CAD build for the part. Positions are in the model's coordinates, mm. A direction names the side the tool comes from. Give positions to 0.01 mm unless a question says otherwise; leave off trailing zeros. Loops run counter-clockwise (first coordinate to the right, second up) from the corner with the lowest first, then second, coordinate; pieces in that order, holes last.
Autodesk Inventor part; units mm, degrees
ref_plane "Arbeitsebene10" through (-35, 70.3553, 70.3553) normal (0, 1, 0) x (1, 0, 0)
ref_plane "Arbeitsebene11" through (-17.5, 90.3553, 53.0624) normal (0, 1, 0) x (1, 0, 0)
ref_plane "Arbeitsebene2" through (-35, 80.3553, 35.7696) normal (0, 1, 0) x (1, 0, 0)
ref_plane "Arbeitsebene10" through (-35, 70.3553, 70.3553) normal (0, 1, 0) x (1, 0, 0)
sketch "Skizze7" plane through (-35, 70.3553, 70.3553) normal (0, 1, 0) x (1, 0, 0)
  circle A0 centre (17.5, 17.2929) radius 11.5
  point P0 (35, 70.3553)
  dimension "d32" = 23
extrude "Achshalter" add sketch "Skizze7" along normal blind 20
ref_plane "Arbeitsebene11" through (-17.5, 90.3553, 53.0624) normal (0, 1, 0) x (1, 0, 0)
sketch "Skizze16" plane through (-17.5, 90.3553, 53.0624) normal (0, 1, 0) x (1, 0, 0)
  circle A0 centre (0, 0) radius 11.5
  arc A1 (2.2, 1.3856) -> (2.2, -1.3856) centre (0, 0) ccw
  line L0 (2.2, 1.3856) -> (2.2, -1.3856)
  point P0 (17.5, 53.0624)
  dimension "d54" = 5.2
  dimension "d55" = 2.2
extrude "Extrusion11" cut sketch "Skizze16" against normal blind 18 contours L0 A1
ref_plane "Arbeitsebene2" through (-35, 80.3553, 35.7696) normal (0, 1, 0) x (1, 0, 0)
sketch "Skizze17" plane through (-35, 80.3553, 35.7696) normal (0, 1, 0) x (1, 0, 0)
  line L0 (30.7802, -4.1446) -> (17.4658, -4.1446)
  line L1 (17.4658, -4.1446) -> (17.4658, -31.1746)
  line L2 (17.4658, -31.1746) -> (30.7802, -31.1746)
  line L3 (30.7802, -31.1746) -> (30.7802, -4.1446)
  point P0 (35, 35.7696)
extrude "Extrusion12" cut sketch "Skizze17" against normal blind 1
ref_plane "Arbeitsebene16" through (-34, 67.3553, 52.8553) normal (0, 0, 1) x (1, 0, 0)
sketch "Skizze18" plane through (-34, 67.3553, 52.8553) normal (0, 0, 1) x (1, 0, 0)
  line L0 (29.7456, 25.5785) -> (16.4577, 25.5785)
  line L1 (16.4577, 25.5785) -> (16.4577, 12.5204)
  line L2 (16.4577, 12.5204) -> (29.7456, 12.5204)
  line L3 (29.7456, 12.5204) -> (29.7456, 25.5785)
  point P0 (34, -67.3553)
extrude "Extrusion13" cut sketch "Skizze18" along normal blind 1 and the other way blind 0.5
ref_plane "Arbeitsebene17" through (-34, 67.3553, 70.3553) normal (0, 0, 1) x (1, 0, 0)
sketch "Skizze19" plane through (-34, 67.3553, 70.3553) normal (0, 0, 1) x (1, 0, 0)
  circle A0 centre (22.3096, 18.1328) radius 1.25
  point P0 (34, -67.3553)
  dimension "d67" = 2.5
extrude "Extrusion14" cut sketch "Skizze19" against normal blind 35
sketch "Skizze24" plane through (-17.5, 70.3553, 53.0624) normal (0, -1, 0) x (1, 0, 0)
  line L0 (-17.5, 17.5) -> (17.5, 17.5)
  line L1 (17.5, 17.5) -> (17.5, -17.5)
  line L2 (17.5, -17.5) -> (-17.5, -17.5)
  line L3 (-17.5, -17.5) -> (-17.5, 17.5)
  point P0 (0, 0)
  point P1 (17.5, -53.0624)
  dimension "d90" = 35
  dimension "d91" = 35
  dimension "d92" = 17.5
  dimension "d93" = 17.5
extrude "Extrusion17" add sketch "Skizze24" along normal blind 5
sketch "Skizze25" plane through (-35, 70.3553, 35.5624) normal (-1, 0, 0) x (0, 0, 1)
  line L0 (35, -5) -> (0, -5)
  line L1 (0, -5) -> (0, -40)
  line L2 (0, -40) -> (35, -40)
  line L3 (35, -40) -> (35, -5)
  point P0 (-35.5624, -70.3553)
  dimension "d96" = 35
  dimension "d97" = 35
extrude "Extrusion18" add sketch "Skizze25" against normal blind 5
fillet "Rundung14" radius 1 1 edges at (-30, 65.3553, 53.0624)
fillet "Rundung15" radius 1 4 edges at (0, 67.8553, 70.5624) (0, 67.8553, 35.5624) (-32.5, 30.3553, 35.5624) (-32.5, 30.3553, 70.5624)
sketch "Skizze26" plane through (-35, 70.3553, 35.5624) normal (-1, 0, 0) x (0, 0, 1)
  line L0 (1, -40) -> (34, -40)
  circle A0 centre (17.5, -22.5) radius 12.5
  point P0 (-35.5624, -70.3553)
  dimension "d102" = 25
  dimension "d103" = 17.5
extrude "Extrusion19" cut sketch "Skizze26" against normal up to surface (5 mm away)
sketch "Skizze27" plane through (-35, 70.3553, 35.5624) normal (-1, 0, 0) x (0, 0, 1)
  circle A0 centre (29, -34) radius 1.4
  circle A1 centre (29, -11) radius 1.4
  circle A2 centre (6, -11) radius 1.4
  circle A3 centre (6, -34) radius 1.4
  point P0 (-35.5624, -70.3553)
  dimension "d106" = 2.8
  dimension "d107" = 2.8
  dimension "d108" = 2.8
  dimension "d109" = 2.8
  dimension "d110" = 23
  dimension "d111" = 23
  dimension "d112" = 23
  dimension "d113" = 23
extrude "Extrusion20" cut sketch "Skizze27" against normal up to surface (5 mm away)
sketch "Skizze28" plane through (-35, 70.3553, 35.5624) normal (-1, 0, 0) x (0, 0, 1)
  circle A0 centre (29, -34) radius 1.4
  circle A1 centre (29, -11) radius 1.4
  circle A2 centre (6, -34) radius 1.4
  circle A3 centre (6, -11) radius 1.4
  circle A4 centre (29, -11) radius 2.5
  circle A5 centre (29, -34) radius 2.5
  circle A6 centre (6, -11) radius 2.5
  circle A7 centre (6, -34) radius 2.5
  point P0 (-35.5624, -70.3553)
  dimension "d116" = 5
  dimension "d117" = 5
  dimension "d118" = 5
  dimension "d119" = 5
extrude "Extrusion21" cut sketch "Skizze28" against normal blind 2
properties part number "zweifach nema v2"
1. Saw through at C-C, the plane x = -8. List the corners of the cut face in (y, z).
Responses:
outline: (65.36, 35.56) - (70.36, 35.56) - (70.36, 46.58) - (79.36, 46.58) - (79.36, 59.54) - (70.36, 59.54) - (70.36, 70.56) - (65.36, 70.56) - close; (80.36, 46.58) - (90.36, 46.58) - (90.36, 52.36) - (80.36, 52.36) - close; (80.36, 53.86) - (90.36, 53.86) - (90.36, 59.54) - (80.36, 59.54) - close
2. Probe line 1 along Z through (x, y) = (-17.5, 84.5); line 2 along Y through (x, z) = (-12.5, 50); line 3 along X through (y, z) = (64, 38). List the from-to ranges inside material, lowest first.
Responses:
line 1: z = 41.56 to 50.46, 55.66 to 64.56
line 2: y = 65.36 to 79.36, 80.36 to 84.54, 86.44 to 90.36
line 3: x = -35 to -30
3. Saw through at D-D, the plane x = -12. List the corners of the cut face in (y, z), and give its area (3 significant figures).
Responses:
outline: (65.36, 35.56) - (70.36, 35.56) - (70.36, 42.96) - (79.36, 42.96) - (79.36, 63.16) - (70.36, 63.16) - (70.36, 70.56) - (65.36, 70.56) - close; (80.36, 42.96) - (84.28, 42.96) - (84.28, 52.36) - (80.36, 52.36) - close; (80.36, 53.86) - (84.28, 53.86) - (84.28, 63.16) - (80.36, 63.16) - close; (86.7, 42.96) - (90.36, 42.96) - (90.36, 52.36) - (86.7, 52.36) - close; (86.7, 53.86) - (90.36, 53.86) - (90.36, 63.16) - (86.7, 63.16) - close
area: 498 mm2
4. Saw through at B-B, the plane y = 44. List the corners of the cut face in (x, z), and give its area (3 significant figures).
Responses:
outline: (-35, 35.56) - (-30, 35.56) - (-30, 41.17) - (-35, 41.17) - close; (-35, 64.95) - (-30, 64.95) - (-30, 70.56) - (-35, 70.56) - close
area: 56.1 mm2
5. Saw through at A-A, the plane z = 48. List the corners of the cut face in (x, y), and give its area (3 significant figures).
Responses:
outline: (-35, 30.36) - (-30, 30.36) - (-30, 36.43) - (-35, 36.43) - close; (-35, 59.28) - (-30, 59.28) - (-30, 64.36) arc R1 cw to (-29, 65.36) - (0, 65.36) - (0, 70.36) - (-7.17, 70.36) - (-7.17, 79.36) - (-17.53, 79.36) - (-17.53, 80.36) - (-7.17, 80.36) - (-7.17, 90.36) - (-27.83, 90.36) - (-27.83, 70.36) - (-35, 70.36) - close; hole circle Ø2.5 at (-11.69, 85.49)
area: 634 mm2
6. Drop flat-ended pins along their axis: pin 1 (1.5 mm diameter, centred on y = 36.5, z = 41.5, fed in from -X); pin 2 (12 mm diameter, centred on x = -13, z = 40, fed in from -Y); pin 3 (7.5 mm diameter, centred on x = -11, y = 85, fed in from +Z); pin 4 (3.5 mm diameter, centred on y = 59.36, z = 41.56, fed in from +X). Give the stop position or say it passes through.
Responses:
pin 1: passes through
pin 2: stops at y = 65.36
pin 3: stops at z = 64.23
pin 4: stops at x = -30
7. Pull direction Y, two halves, no side cores. Call faces 1 (the face through (-10, 85, 53.855)), 2 (the face through (-34.014, 61.045, 62.72)), 3 (the face through (-33, 35, 66)), 4 (the face through (-18, 72.355, 53)): released by +Y, released by -Y, zero draft, split by the parting line, or undercut.
Responses:
face 1: zero draft
face 2: undercut
face 3: undercut
face 4: released by +Y
8. Tool access for faces 5 (the face through (-30, 44, 41)), 6 (the face through (-15.3, 76, 53)), 7 (the face through (-34.01, 34.83, 62.58)): list every direction of +Z, -Z, +X, -X, +Y, -Y with a clear straight run to the whole face (end or side of a thin tool).
Responses:
face 5: +Z, -Z, +X, -Y
face 6: +Y
face 7: -X
